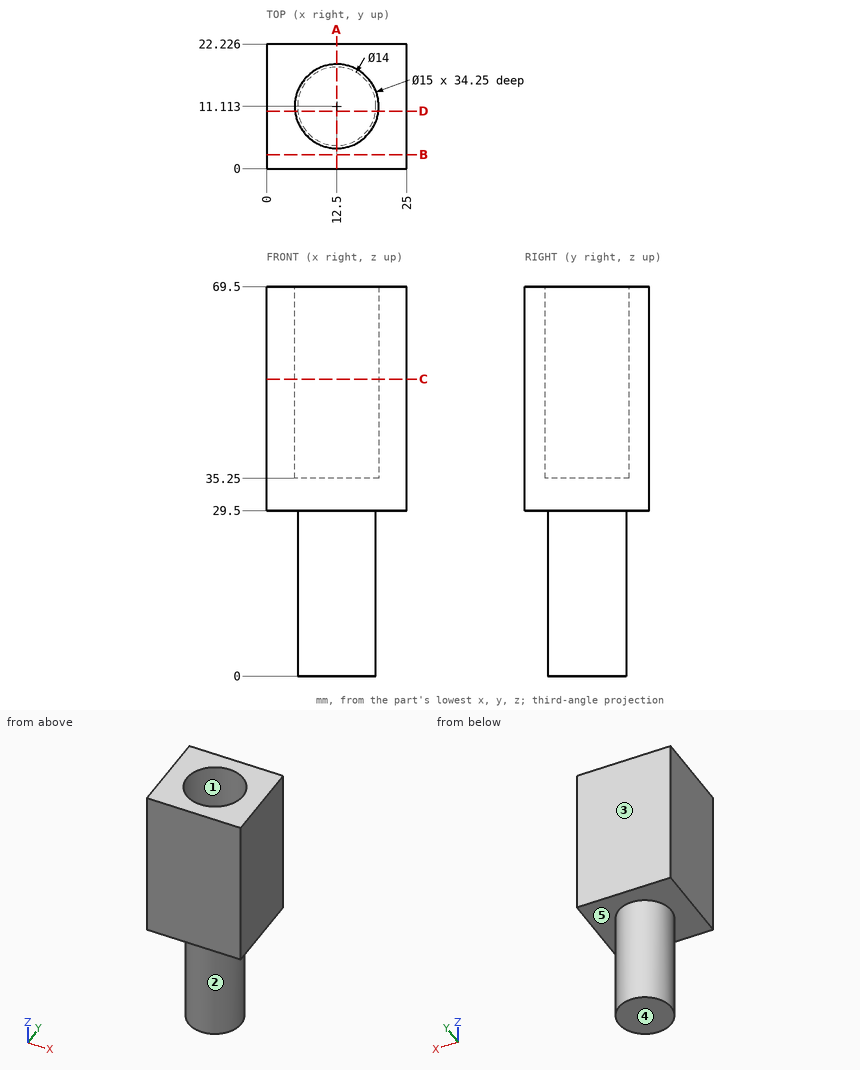
Study the drawing (mm; zero at the part's minimum x, y, z) and answer. A direction names the side the tool comes from. Round coordinates to 2 decimals unless told otherwise and drop trailing zeros. Write each loop counter-clockwise with the first axis right and the second up, starting at its lowest first coordinate (ties: lowest second). Pieces come first, ordered by that corner, then holes. Notation, with made-up numbers: (59, 43.25) -> (74, 43.25) arc R29 cw to (74, 63.25) -> close; hole circle Ø2 at (6, -16.5). An arc over 180 degrees is marked (long way). Answer as CSV lines item,"result". Start each with the question number.
(1) The part is cut by section B-B, the plane y = 2.5. Give the vertices of the cut face in (x, z), then the cut area to 3 significant figures.
(2) The part is cut by section C-C, the plane z = 53. Give the vertices of the cut face in (x, y), then the cut area to 3 significant figures.
(3) The part is cut by section A-A, the plane x = 12.5. Give the vertices of the cut face in (y, z).
(4) Find the intervals of material crossed by probe 1 along Y at (x, z) = (12.5, 59); probe 2 along X at (y, z) = (11.25, 67); probe 3 along Z at (x, y) = (15.75, 11.25), in increasing order.
(5) A tool of negligible diameter and unlimited length cuts with its end or side. For the marked faces 4 and 5, from which of +Z, -Z, +X, -X, +Y, -Y can it reach the whole face along a straight path? Write none if from no direction.
(6) Each of these flat-tipped pins is pushed along its axis until it touches: pin 1 (3 mm diameter, centred on x = 16.5, z = 16.5, fed in from -Y) (1 decimal); pin 2 (1 mm diameter, centred on x = 4, z = 11, fed in from -Y); pin 3 (1 mm diameter, centred on x = 4, y = 11, fed in from -Z); pin 4 (4.5 mm diameter, centred on x = 15.5, y = 12, fed in from +Z). Where does it stop, or does it pass through?
(7) The part is cut by section D-D, the plane y = 10.25. Give the vertices of the cut face in (x, z).
(8) The mould has two halves that part along X. Classify the marked faces 1, 2 and 3: +X half, -X half, draft (parallel to the pull), parting line (faces both ways), or undercut.
Output values:
1,outline,"(0, 29.5) -> (25, 29.5) -> (25, 69.5) -> (0, 69.5) -> close"
1,area,"1,000 mm²"
2,outline,"(0, 0) -> (25, 0) -> (25, 22.23) -> (0, 22.23) -> close; hole circle Ø15 at (12.5, 11.11)"
2,area,"379 mm²"
3,outline,"(0, 29.5) -> (4.11, 29.5) -> (4.11, 0) -> (18.11, 0) -> (18.11, 29.5) -> (22.23, 29.5) -> (22.23, 69.5) -> (18.61, 69.5) -> (18.61, 35.25) -> (3.61, 35.25) -> (3.61, 69.5) -> (0, 69.5) -> close"
4,probe 1,"y = 0 to 3.61, 18.61 to 22.23"
4,probe 2,"x = 0 to 5, 20 to 25"
4,probe 3,"z = 0 to 35.25"
5,face 4,"-Z, +X, -X, +Y, -Y"
5,face 5,"-Z"
6,pin 1,"stops at y = 4.6"
6,pin 2,"passes through"
6,pin 3,"stops at z = 29.5"
6,pin 4,"stops at z = 35.25"
7,outline,"(0, 29.5) -> (5.55, 29.5) -> (5.55, 0) -> (19.45, 0) -> (19.45, 29.5) -> (25, 29.5) -> (25, 69.5) -> (19.95, 69.5) -> (19.95, 35.25) -> (5.05, 35.25) -> (5.05, 69.5) -> (0, 69.5) -> close"
8,face 1,"undercut"
8,face 2,"parting line"
8,face 3,"draft"
